Here's how the part is built. I have some questions about the finished solid (model axes, mm). A direction names the side the tool comes from. Round coordinates to 2 decimals unless told otherwise and drop trailing zeros. Order: outer loops, then holes, each group sorted by start corner. A loop starts at its lowest first (then second) coordinate and runs counter-clockwise, first axis right, second up.
```python
from build123d import *

# Parameters (mm, degrees)
BOSS_EXTRUDE1_DEPTH = 30
SKETCH2_R           = 4.4
CUT_EXTRUDE1_DEPTH  = 97.608495293
SKETCH4_W           = 26
SKETCH4_H           = 53.255509589
CUT_EXTRUDE2_DEPTH  = 40


with BuildPart() as part:
    # Sketch1 → Boss-Extrude1 (new body)
    with BuildSketch(Plane.XY):
        with BuildLine():
            Line((-41.88810428, 5.785), (12.276322135, 15.335649772))
            ThreePointArc((12.276322135, 15.335649772), (23.057327156, 49.569411506), (57.276322135, 60.397194952))
            ThreePointArc((57.276322135, 60.397194952), (59.00041024, 58.767721176), (58.177057872, 56.542916587))
            Line((58.177057872, 56.542916587), (50.110478485, 50.632730719))
            ThreePointArc((50.110478485, 50.632730719), (47.703320965, 47.797119103), (46.838627179, 44.179467209))
            Line((46.838627179, 44.179467209), (46.838627179, 19.179467209))
            ThreePointArc((46.838627179, 19.179467209), (48.595986492, 14.936826522), (52.838627179, 13.179467209))
            Line((52.838627179, 13.179467209), (59.088627179, 13.179467209))
            ThreePointArc((59.088627179, 13.179467209), (68.507642402, 5.328734817), (62.482043199, -5.350403777))
            Line((62.482043199, -5.350403777), (28.173137316, -18.352594225))
            ThreePointArc((28.173137316, -18.352594225), (21.856973189, -19.111848957), (15.915778413, -16.837513523))
            ThreePointArc((15.915778413, -16.837513523), (14.177787103, -15.888509343), (12.276322135, -15.335649772))
            Line((12.276322135, -15.335649772), (-41.88810428, -5.785))
            Line((-41.88810428, -5.785), (-41.88810428, 5.785))
        make_face()
    extrude(amount=BOSS_EXTRUDE1_DEPTH)

    # Sketch2 → Cut-Extrude1 (cut, through all)
    with BuildSketch(Plane.XY.offset(30)):
        with Locations((59.088627179, 3.603809847)):
            Circle(SKETCH2_R)
    extrude(amount=-CUT_EXTRUDE1_DEPTH, mode=Mode.SUBTRACT)

    # Sketch4 → Cut-Extrude2 (cut)
    with BuildSketch(Plane(origin=(70, 0, 0), x_dir=(0, 0, -1), z_dir=(1, 0, 0))):
        with Locations((-15, 24.841006249)):
            Rectangle(SKETCH4_W, SKETCH4_H)
    extrude(amount=-CUT_EXTRUDE2_DEPTH, mode=Mode.SUBTRACT)


solid = part.part
```
1. If we section it at C-C, the plane y = 27.5: Write out the boundary of the cut face in (x, z), and give its area (3 significant figures).
Evaluation:
outline: (12.06, 0) - (46.84, 0) - (46.84, 2) - (30, 2) - (30, 28) - (46.84, 28) - (46.84, 30) - (12.06, 30) - close
area: 605 mm2
2. If we mould it in two halves opening along Y, with no side actions, what happens to faces 4 (the flat face through (14, 13, 0)), 5 (the cylindrical face through (21.946, -19.123, 14.79)), 6 (the cylindrical face through (48.55, 14.984, 28.986)), 7 (the flat face through (41, 19, 2))? For each: released by +Y, released by -Y, zero draft, split by the parting line, or undercut.
Evaluation:
face 4: zero draft
face 5: released by -Y
face 6: undercut
face 7: undercut
3. On a 3-axis mill with a long thin cutter (end or side, diameter ignored), from which of +Z, -Z, +X, -X, +Y, -Y can I reach the whole of each face in a straight line? I mean faces 1 (the flat face through (30, 25, 15)), 2 (the flat face through (-14.427, -10.627, 14.79)), 3 (the cylindrical face through (48.55, 14.984, 0.986)). Say none if no direction works.
Evaluation:
face 1: +X
face 2: +Z, -Z, -X, -Y
face 3: +Z, -Z, +X
4. If we section it at B-B, the plane x = 41: Write out the boundary of the cut face in (y, z).
Evaluation:
outline: (-13.49, 0) - (59.78, 0) - (59.78, 30) - (-13.49, 30) - close; hole (-1.79, 2) - (51.47, 2) - (51.47, 28) - (-1.79, 28) - close
5. If we section it at D-D, the plane x = 5: Write out the boundary of the cut face in (y, z), and give its area (3 significant figures).
Evaluation:
outline: (-14.05, 0) - (14.05, 0) - (14.05, 30) - (-14.05, 30) - close
area: 843 mm2
6. I need wall thicknesses on probe 1 along Z at (x, y) = (33, 28); probe 2 along X at (y, z) = (38.5, 11.5); probe 3 along Y at (x, z) = (43, 8.25). Which ranges of each line are inside material? Lowest first, please.
Evaluation:
probe 1: z = 0 to 2, 28 to 30
probe 2: x = 15.32 to 30
probe 3: y = -12.73 to -1.79, 51.47 to 60.23
7. I'm going to push flat-ended pins straight in: P1, Ø4, axis at x = 6.5, z = 22.5, coming from the +Y side; P2, Ø1.6, axis at y = 32.5, z = 29, coming from the +X side; P3, Ø12, axis at x = -5, z = 20.5, coming from the +Y side; P4, Ø12, axis at x = 48, y = 11.5, coming from the -Z side. Where does each tip first touch, or does it pass through?
Evaluation:
P1: stops at y = 14.67
P2: stops at x = 46.84
P3: stops at y = 13.35
P4: stops at z = 0
